Autodesk Fusion 360 part; units mm, degrees
sketch "Sketch1" plane through (0, 0, 0) normal (0, 0, 1) x (1, 0, 0) in component "boiler"
  line L0 (38.8029, -38.8029) -> (54.8756, 0)
  line L1 (54.8756, 0) -> (38.8029, 38.8029)
  line L2 (38.8029, 38.8029) -> (0, 54.8756)
  line L3 (0, 54.8756) -> (-38.8029, 38.8029)
  line L4 (-38.8029, 38.8029) -> (-54.8756, 0)
  line L5 (-54.8756, 0) -> (-38.8029, -38.8029)
  line L6 (-38.8029, -38.8029) -> (0, -54.8756)
  line L7 (0, -54.8756) -> (38.8029, -38.8029)
  line L8 (0, 0) -> (0, -54.8756) construction
  dimension "d1" = 42
extrude "Extrude1" add sketch "Sketch1" along normal blind 80 draft -8 in component "boiler"
sketch "Sketch2" plane through (-19.0257, -45.9321, 6.9872) normal (-0.379, -0.9149, 0.1392) x (0.9239, -0.3827, 0) in component "boiler"
  line L0 (16.3429, 73.7303) -> (-16.3429, 73.7303)
  line L1 (-16.3429, 73.7303) -> (-21, -7.0559)
  line L2 (-21, -7.0559) -> (21, -7.0559)
  line L3 (21, -7.0559) -> (16.3429, 73.7303)
sketch "Sketch3" plane through (19.0257, -45.9321, 6.9872) normal (0.379, -0.9149, 0.1392) x (0.9239, 0.3827, 0) in component "boiler"
  line L0 (16.3429, 73.7303) -> (-16.3429, 73.7303)
  line L1 (-16.3429, 73.7303) -> (-21, -7.0559)
  line L2 (-21, -7.0559) -> (21, -7.0559)
  line L3 (21, -7.0559) -> (16.3429, 73.7303)
sketch "Sketch1 (2)" plane through (0, 0, 0) normal (1, 0, 0) x (0, 1, 0)
sketch "Sketch5" plane through (0, 0, 0) normal (1, 0, 0) x (0, 1, 0) in component "boiler"
  line L0 (-65, 0) -> (-57, 9)
  line L1 (-57, 9) -> (-39, 0)
  line L2 (-39, 0) -> (-65, 0)
revolve "Revolve1" cut sketch "Sketch5" angle 360 about axis through (0, 0, 1.75) along (0, 0, 1) in component "boiler"
sketch "Sketch2 (2)" plane through (0, 0, 0) normal (0, 1, 0) x (1, 0, 0)
  line L0 (-53.7535, -7.3767) -> (-42.706, -80)
  line L1 (-30.1977, -80) -> (-42.706, -80)
  line L2 (-36.4519, -80) -> (-43.9675, -71.7075)
revolve "Revolve2" cut sketch "Sketch2 (2)" angle 360 about axis through (0, 0, 1.75) along (0, 0, 1) in component "boiler"
extrude "Extrude2" add 1 faces at (9.3758, -5.1542, 80) along direction (0, 0, 1) blind 15 in component "boiler"
fillet "Fillet1" radius 6 1 edges at (33.9851, 13.1816, 80) in component "boiler"
shell "Shell1" thickness 2 removed faces 1 at (9.3758, -5.1542, 95) in component "boiler"
component "boiler" placed x (1, 0, 0) y (0, 1, 0) z (0, 0, 1) at (0, 0, 0)
The model under review builds one solid part; all positions refer to its coordinate system, in mm. A direction names the side the tool comes from. Round coordinates to 2 decimals unless told otherwise and drop trailing zeros. Order: outer loops, then holes, each group sorted by start corner. A loop starts at its lowest first (then second) coordinate and runs counter-clockwise, first axis right, second up. Notation, with made-up numbers: (52, -36) -> (69, -36) arc R27 ccw to (69, -14) -> close; hole circle Ø8 at (66, 45). An arc over 180 degrees is marked (long way). Write item = value, one per line. Start each with the question number.
Item 1: Clearance check with flat-ended pins moving along their axes: pin 1 Ø5 at (y, z) = (29.5, 32.5) entering from -X; pin 2 Ø12 at (x, y) = (32.5, -42.5) entering from -Z; pin 3 Ø3 at (x, z) = (-10.5, 82.5) entering from -Y. State where each tip first meets the part, or that it passes through.
Item 2: Consider section A-A on z = 52. Write out the cut boundary in (x, y), plus the area to 3 significant figures.
Item 3: Mouldability with a two-part tool opening along Y and no side actions: class faces 1 (the face through (26.98, 29.42, 0.46)), 2 (the face through (-16.2, 39.83, 40.42)), 3 (the face through (-16.97, 41.72, 40.28)) as released by +Y, released by -Y, zero draft, split by the parting line, or undercut.
Item 4: Consider section B-B on z = 28.5. Write out the cut boundary in (x, y).
Item 5: For faces 4 (the face through (-18.52, 29.05, 88.57)), 5 (the face through (-1, 1, 2)), 6 (the face through (-41.72, -16.97, 40.28)), list the 3-axis set-ups (+Z, -Z, +X, -X, +Y, -Y) from which the entire face can be reached by the end or side of a thin tool; tool diameter is ignored.
Item 6: For line 1 along Y through (x, z) = (0, 86), list the stretches that pass through material, from the lowest coordinate up.
Conclusion:
q1.pin_1 = -38.82
q1.pin_2 = 4.25
q1.pin_3 = -35.32
q2.outline = (-46.97, 0) -> (-33.21, -33.21) -> (0, -46.97) -> (33.21, -33.21) -> (46.97, 0) -> (33.21, 33.21) -> (0, 46.97) -> (-33.21, 33.21) -> close; hole (-44.78, 0) -> (-31.66, -31.66) -> (0, -44.78) -> (31.66, -31.66) -> (44.78, 0) -> (31.66, 31.66) -> (0, 44.78) -> (-31.66, 31.66) -> close
q2.area = 567 mm2
q3.face_1 = split by the parting line
q3.face_2 = undercut
q3.face_3 = released by +Y
q4.outline = (-50.54, 0) -> (-35.74, -35.74) -> (0, -50.54) -> (35.74, -35.74) -> (50.54, 0) -> (35.74, 35.74) -> (0, 50.54) -> (-35.74, 35.74) -> close; hole (-48.35, 0) -> (-34.19, -34.19) -> (0, -48.35) -> (34.19, -34.19) -> (48.35, 0) -> (34.19, 34.19) -> (0, 48.35) -> (-34.19, 34.19) -> close
q5.face_4 = +Z
q5.face_5 = none
q5.face_6 = +Z, -X, -Y
q6.line_1 = -36.45 to -34.45, 34.45 to 36.45
